The model under review builds one solid part; all positions refer to its coordinate system, in mm. Face numbers are marked on the shaded views. A direction names the side the tool comes from. Round coordinates to 2 decimals unless told otherwise and drop trailing zeros. Order: outer loops, then holes, each group sorted by start corner. A loop starts at its lowest first (then second) coordinate and runs counter-clockwise, first axis right, second up. Notation, with made-up numbers: (17, -31) - (47, -31) arc R17 ccw to (47, -9) - close; hole circle Ø2 at (24.25, -22.75). An arc over 180 degrees is marked (long way). One line per question, with ' | ' between items. Start each with the question number.
Item 1: Draft analysis for pull direction Y (two halves, no side actions). For the marked faces 4, 5, 6 and 7, state which applies: +Y half, -Y half, draft (parallel to the pull), parting line (faces both ways), or undercut.
Item 2: Tool access review of the marked faces 1, 2 and 3: name each direction out of +Z, -Z, +X, -X, +Y, -Y from which nothing blocks a thin tool from reaching the whole face with its end or side.
Item 3: Add section A-A on x = 11.5. State the section outline as (y, z) points.
Item 4: Add section B-B on y = 1.75. State the section outline as (x, z) points (3 decimals), and give its area (3 significant figures).
Item 5: Add section D-D on y = -5.5. State the section outline as (x, z) points, and give its area (3 significant figures).
Item 6: For L1, parallel to Y at x = 4.5, z = -1.25; L2, parallel to Z at x = 0, y = -12.5; L3, parallel to Z at x = 0, y = 2.9 (3 decimals), list the stretches that pass through material, from the lowest coordinate up. Write a range as [from, to].
Item 7: Add section C-C on x = 0. State how many separate pieces and enclosed holes the cut face has, and give its area (3 significant figures).
Item 8: Insertion check: pin 1 Ø5.5 at (x, z) = (30.5, 1.5) entering from +Y; pin 2 Ø5.5 at (x, z) = (30.5, -1.5) entering from -Y; pin 3 Ø1.2 at (y, z) = (-1.5, 1) entering from +X. Each pin has a flat end and moves straight along its axis. Give the tip position at first contact, or say it passes through.
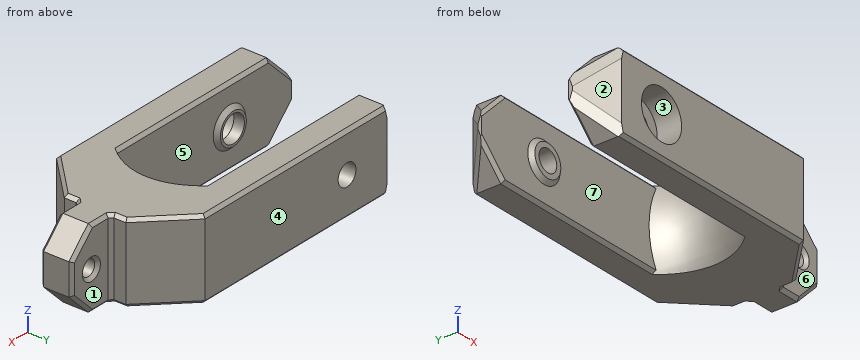
from build123d import *

# Parameters (mm, degrees)
BOSS_EXTRUDE1_DEPTH      = 5
BOSS_EXTRUDE1_DEPTH_BACK = 5
CUT_EXTRUDE1_DEPTH       = 34.669323141
CUT_EXTRUDE1_DEPTH_BACK  = 34.669323141
SKETCH2_R                = 1.375
CUT_EXTRUDE2_REACH       = 35.669
SKETCH3_R                = 1.7
SKETCH4_R                = 3.1
CUT_EXTRUDE3_DEPTH       = 3.1
CHAMFER1_SIZE            = 3.43398
CUT_EXTRUDE4_START       = -5
CUT_EXTRUDE4_DEPTH       = 10
CHAMFER2_SIZE            = 0.4
CHAMFER3_SIZE            = 0.4
CHAMFER3_EDGE_2_SIZE     = 0.4
CHAMFER3_EDGE_2_SIZE2    = 1.092820323
CHAMFER3_EDGE_3_SIZE     = 0.4
CHAMFER3_EDGE_3_SIZE2    = 1.092820323
CHAMFER3_EDGE_4_SIZE     = 0.4
CHAMFER3_EDGE_5_SIZE     = 0.4
CHAMFER3_EDGE_6_SIZE     = 0.4
CHAMFER3_EDGE_7_SIZE     = 0.4
CHAMFER3_EDGE_7_SIZE2    = 1.092820323
CHAMFER3_EDGE_8_SIZE     = 0.4
CHAMFER3_EDGE_8_SIZE2    = 1.092820323
SKETCH9_W                = 10
SKETCH9_H                = 4
BOSS_EXTRUDE3_DEPTH      = 6
CUT_EXTRUDE5_REACH       = 37.687
SKETCH10_R               = 1
CHAMFER4_SIZE            = 0.4
CHAMFER5_SIZE            = 3
CHAMFER6_SIZE            = 0.4
MOVE_FACE1_OUTLINE_R     = 1.7
MOVE_FACE1_OUTLINE_R_2   = 1.375
MOVE_FACE1_DEPTH         = 0.5


# Read off the part's stored shape, not the designer's step: Move Face1
with BuildPart() as part:
    # Sketch1 → Boss-Extrude1 (new, two sides: drawn at the far end of the back side and taken through both)
    with BuildSketch(Plane.XY.offset(-BOSS_EXTRUDE1_DEPTH_BACK)):
        Polygon((27.433981132, -1.092317068), (21.907682932, 4.433981132), (-6.166018868, 4.433981132), (-9.6, 1), (-9.6, 0.5), (11.1, 0.5), (11.1, -10.5), (-9.6, -10.5), (-9.6, -11), (-6.166018868, -14.433981132), (21.907682932, -14.433981132), (27.433981132, -8.907682932), align=None)
    extrude(amount=BOSS_EXTRUDE1_DEPTH + BOSS_EXTRUDE1_DEPTH_BACK)

    # Sketch2 → Cut-Extrude1 (cut, two sides: drawn at the far end of the back side and taken through both)
    with BuildSketch(Plane.XZ.offset(14.433981132).offset(-CUT_EXTRUDE1_DEPTH_BACK)):
        Circle(SKETCH2_R)
    extrude(amount=CUT_EXTRUDE1_DEPTH + CUT_EXTRUDE1_DEPTH_BACK, mode=Mode.SUBTRACT)

    # Sketch3 → Cut-Extrude2 (cut, up to next)
    with BuildSketch(Plane.XZ.offset(14.433981132), mode=Mode.PRIVATE) as cut_extrude2_sk1:
        Circle(SKETCH3_R)
    cut_extrude2_tool1 = extrude(cut_extrude2_sk1.sketch, amount=-CUT_EXTRUDE2_REACH, mode=Mode.PRIVATE) & part.part
    add(cut_extrude2_tool1.solids().sort_by_distance((0, -14.433981, 0))[0], mode=Mode.SUBTRACT)

    # Sketch4 → Cut-Extrude3 (cut)
    with BuildSketch(Plane.XZ.offset(14.433981132)):
        Circle(SKETCH4_R)
    extrude(amount=-CUT_EXTRUDE3_DEPTH, mode=Mode.SUBTRACT)

    # Sketch5 → Revolve1 (revolve)
    with BuildSketch(Plane.XY, mode=Mode.PRIVATE) as revolve1_sk:
        Polygon((-1.7, -10.5), (-2.5, -10.5), (-2, -10), (-1.7, -10), align=None)
    revolve1 = revolve(revolve1_sk.sketch.rotate(Axis((0, 4.433981132, 0), (0, -1, 0)), 180), axis=Axis((0, 4.433981132, 0), (0, -1, 0)))

    # Mirror1: Revolve1 across plane
    add(revolve1.mirror(Plane(origin=(0, -5, 0), x_dir=(0, 0, 1), z_dir=(0, -1, 0))))

    # Chamfer1
    chamfer1_edges = [part.edges().sort_by_distance(p)[0] for p in [
        (-9.6, 0.75, 5),
        (-9.6, 0.75, -5),
        (-9.6, -10.75, -5),
        (-9.6, -10.75, 5),
    ]]
    chamfer(chamfer1_edges, length=CHAMFER1_SIZE)

    # Sketch7 → Cut-Extrude4 (cut)
    with BuildSketch(Plane.XY.offset(CUT_EXTRUDE4_START)):
        with BuildLine():
            Line((11.1, 0.5), (11.1, -10.5))
            Line((11.1, -10.5), (16.230873726, -10.5))
            ThreePointArc((16.230873726, -10.5), (18, -5), (16.230873726, 0.5))
            Line((16.230873726, 0.5), (11.1, 0.5))
        make_face()
    extrude(amount=CUT_EXTRUDE4_DEPTH, mode=Mode.SUBTRACT)

    # Sketch7<2> → Cut-Revolve3 (revolve, cut)
    with BuildSketch(Plane.XY):
        with BuildLine():
            Line((11.1, 0.5), (11.1, -10.5))
            Line((11.1, -10.5), (16.230873726, -10.5))
            ThreePointArc((16.230873726, -10.5), (18, -5), (16.230873726, 0.5))
            Line((16.230873726, 0.5), (11.1, 0.5))
        make_face()
    revolve(axis=Axis((26.566018868, 5.861349866, 0), (0, -1, 0)), mode=Mode.SUBTRACT)

    # Chamfer2
    chamfer2_edges = [part.edges().sort_by_distance(p)[0] for p in [
        (5.677410985, -10.5, -5),
        (7.870832032, -14.433981132, -5),
        (24.670832032, -11.670832032, -5),
        (5.677410985, -10.5, 5),
        (7.870832032, -14.433981132, 5),
        (24.670832032, -11.670832032, 5),
        (24.670832032, 1.670832032, 5),
        (24.670832032, 1.670832032, -5),
        (7.870832032, 4.433981132, 5),
        (7.870832032, 4.433981132, -5),
        (5.677410985, 0.5, 5),
        (5.677410985, 0.5, -5),
    ]]
    chamfer(chamfer2_edges, length=CHAMFER2_SIZE)

    # Chamfer3
    chamfer3_edges = [part.edges().sort_by_distance(p)[0] for p in [
        (-8.08301, 0.5, 3.08301),
    ]]
    chamfer(chamfer3_edges, length=CHAMFER3_SIZE)

    # Chamfer3 edge 2
    chamfer3_edge_2_edges = [part.edges().sort_by_distance(p)[0] for p in [
        (-7.983009717, 2.616990283, 3.183010283),
    ]]
    chamfer3_edge_2_side = [part.faces().sort_by_distance(p)[0] for p in [
        (-7.458377293, 1.830066089, 3.707642707),
    ]]
    chamfer(chamfer3_edge_2_edges, length=CHAMFER3_EDGE_2_SIZE, length2=CHAMFER3_EDGE_2_SIZE2, reference=chamfer3_edge_2_side[0])

    # Chamfer3 edge 3
    chamfer3_edge_3_edges = [part.edges().sort_by_distance(p)[0] for p in [
        (-7.983009717, 2.616990283, -3.183010283),
    ]]
    chamfer3_edge_3_side = [part.faces().sort_by_distance(p)[0] for p in [
        (-7.458377293, 1.830066089, -3.707642707),
    ]]
    chamfer(chamfer3_edge_3_edges, length=CHAMFER3_EDGE_3_SIZE, length2=CHAMFER3_EDGE_3_SIZE2, reference=chamfer3_edge_3_side[0])

    # Chamfer3 edge 4
    chamfer3_edge_4_edges = [part.edges().sort_by_distance(p)[0] for p in [
        (-8.08301, 0.5, -3.08301),
    ]]
    chamfer(chamfer3_edge_4_edges, length=CHAMFER3_EDGE_4_SIZE)

    # Chamfer3 edge 5
    chamfer3_edge_5_edges = [part.edges().sort_by_distance(p)[0] for p in [
        (-8.08301, -10.5, 3.08301),
    ]]
    chamfer(chamfer3_edge_5_edges, length=CHAMFER3_EDGE_5_SIZE)

    # Chamfer3 edge 6
    chamfer3_edge_6_edges = [part.edges().sort_by_distance(p)[0] for p in [
        (-8.08301, -10.5, -3.08301),
    ]]
    chamfer(chamfer3_edge_6_edges, length=CHAMFER3_EDGE_6_SIZE)

    # Chamfer3 edge 7
    chamfer3_edge_7_edges = [part.edges().sort_by_distance(p)[0] for p in [
        (-7.983009717, -12.616990283, 3.183010283),
    ]]
    chamfer3_edge_7_side = [part.faces().sort_by_distance(p)[0] for p in [
        (-7.458377293, -11.830066089, 3.707642707),
    ]]
    chamfer(chamfer3_edge_7_edges, length=CHAMFER3_EDGE_7_SIZE, length2=CHAMFER3_EDGE_7_SIZE2, reference=chamfer3_edge_7_side[0])

    # Chamfer3 edge 8
    chamfer3_edge_8_edges = [part.edges().sort_by_distance(p)[0] for p in [
        (-7.983009717, -12.616990283, -3.183010283),
    ]]
    chamfer3_edge_8_side = [part.faces().sort_by_distance(p)[0] for p in [
        (-7.458377293, -11.830066089, -3.707642707),
    ]]
    chamfer(chamfer3_edge_8_edges, length=CHAMFER3_EDGE_8_SIZE, length2=CHAMFER3_EDGE_8_SIZE2, reference=chamfer3_edge_8_side[0])

    # Sketch9 → Boss-Extrude3 (add)
    with BuildSketch(Plane(origin=(27.433981132, 0, 0), x_dir=(0, 0, -1), z_dir=(1, 0, 0))):
        with Locations((0, -5)):
            Rectangle(SKETCH9_W, SKETCH9_H)
    extrude(amount=BOSS_EXTRUDE3_DEPTH)

    # Sketch10 → Cut-Extrude5 (cut, up to next)
    with BuildSketch(Plane(origin=(0, -3, 0), x_dir=(1, 0, 0), z_dir=(0, 1, 0)), mode=Mode.PRIVATE) as cut_extrude5_sk1:
        with Locations(Location((30.433981132, 0, 0), (0, 0, 270))):
            Circle(SKETCH10_R)
    cut_extrude5_tool1 = extrude(cut_extrude5_sk1.sketch, amount=-CUT_EXTRUDE5_REACH, mode=Mode.PRIVATE) & part.part
    add(cut_extrude5_tool1.solids().sort_by_distance((30.433981, -3, 0))[0], mode=Mode.SUBTRACT)

    # Chamfer4
    chamfer4_edges = [part.edges().sort_by_distance(p)[0] for p in [
        (27.433981132, -3, 0),
        (27.433981132, -7, 0),
    ]]
    chamfer(chamfer4_edges, length=CHAMFER4_SIZE)

    # Chamfer5
    chamfer5_edges = [part.edges().sort_by_distance(p)[0] for p in [
        (33.433981132, -5, -5),
        (33.433981132, -5, 5),
    ]]
    chamfer(chamfer5_edges, length=CHAMFER5_SIZE)

    # Chamfer6
    chamfer6_edges = [part.edges().sort_by_distance(p)[0] for p in [
        (30.433981132, -3, -1),
        (30.433981132, -7, -1),
        (27.433981132, -7.870998754, 5),
        (27.633981132, -7.2, 5),
        (27.633981132, -7.2, -5),
        (29.133981132, -7, 5),
        (31.933981132, -7, 3.5),
        (33.433981132, -7, 0),
        (31.933981132, -7, -3.5),
        (27.433981132, -7.870998754, -5),
        (29.133981132, -7, -5),
        (27.433981132, -2.129001246, 5),
        (27.633981132, -2.8, -5),
        (27.633981132, -2.8, 5),
        (29.133981132, -3, 5),
        (31.933981132, -3, 3.5),
        (33.433981132, -3, 0),
        (31.933981132, -3, -3.5),
        (29.133981132, -3, -5),
        (27.433981132, -2.129001246, -5),
    ]]
    chamfer(chamfer6_edges, length=CHAMFER6_SIZE)

    # Move Face1 outline → Move Face1 (add)
    with BuildSketch(Plane(origin=(0, 0, 0), x_dir=(1, 0, 0), z_dir=(0, 1, 0))):
        Circle(MOVE_FACE1_OUTLINE_R)
        Circle(MOVE_FACE1_OUTLINE_R_2, mode=Mode.SUBTRACT)
    extrude(amount=MOVE_FACE1_DEPTH)


solid = part.part
Determined:
1) face 4: +Y half | face 5: undercut | face 6: -Y half | face 7: undercut
2) face 1: +Z, -Z, +X, +Y | face 2: +Z, -Z, -X, -Y | face 3: -Y
3) outline: (-14.43, -4.6) - (-14.03, -5) - (-10.9, -5) - (-10.5, -4.6) - (-10.5, 4.6) - (-10.9, 5) - (-14.03, 5) - (-14.43, 4.6) - close; (0.5, -4.6) - (0.9, -5) - (4.03, -5) - (4.43, -4.6) - (4.43, 4.6) - (4.03, 5) - (0.9, 5) - (0.5, 4.6) - close
4) outline: (-8.85, -0.978) - (-8.36, -2.806) - (-6.166, -5) - (24.026, -5) - (24.592, -4.6) - (24.592, 4.6) - (24.026, 5) - (-6.166, 5) - (-8.36, 2.806) - (-8.85, 0.978) - close; hole circle Ø2.75 at (0, 0) | area: 320 mm2
5) outline: (19.59, -5) - (30.43, -5) - (33.43, -2) - (33.43, 2) - (30.43, 5) - (19.59, 5) arc R8.58 ccw to start; hole circle Ø2 at (30.43, 0) | area: 137 mm2
6) L1: [-14.43, -10.5], [0.5, 4.43] | L2: [-5, -3.1], [3.1, 5] | L3: [-5, -1.375], [1.375, 5]
7) separate pieces: 4 | enclosed holes: 0 | area: 46.6 mm2
8) pin 1: y = -2.92 | pin 2: y = -7.08 | pin 3: x = 27.43
